from build123d import *

# Parameters (mm, degrees)
SKETCH1_W             = 50.8
SKETCH1_H             = 50.8
BOSS_EXTRUDE1_DEPTH   = 12.7
F_8_CLEARANCE_HOLE1_D = 4.4958
SKETCH5_R             = 13.208
CUT_EXTRUDE1_DEPTH    = 1.5875
SKETCH6_R             = 3.81
CUT_EXTRUDE2_DEPTH    = 39.1
SKETCH10_R            = 6.858
CUT_EXTRUDE3_DEPTH    = 3.175
CUT_EXTRUDE4_START    = -5.334
SKETCH11_R            = 6.858
CUT_EXTRUDE4_DEPTH    = 5.334
SKETCH12_R            = 1.016
CUT_EXTRUDE5_DEPTH    = 19.05
CUT_EXTRUDE6_START    = -19.05
SKETCH13_R            = 1.016
CUT_EXTRUDE6_DEPTH    = 19.05


with BuildPart() as part:
    # Sketch1 → Boss-Extrude1 (new body)
    with BuildSketch(Plane(origin=(0, 0, 0), x_dir=(1, 0, 0), z_dir=(0, 1, 0))):
        Rectangle(SKETCH1_W, SKETCH1_H)
    extrude(amount=BOSS_EXTRUDE1_DEPTH)

    # #8 Clearance Hole1 (through all)
    with Locations(Plane(origin=(0, 12.7, 0), x_dir=(1, 0, 0), z_dir=(0, 1, 0))):
        with Locations((-19.05, -19.05), (-19.05, 19.05), (19.05, 19.05), (19.05, -19.05)):
            Hole(F_8_CLEARANCE_HOLE1_D / 2)

    # Sketch5 → Cut-Extrude1 (cut)
    with BuildSketch(Plane(origin=(0, 12.7, 0), x_dir=(1, 0, 0), z_dir=(0, 1, 0))):
        with Locations(Location((0, 0, 0), (0, 0, 270))):
            Circle(SKETCH5_R)
    extrude(amount=-CUT_EXTRUDE1_DEPTH, mode=Mode.SUBTRACT)

    # Sketch6 → Cut-Extrude2 (cut, through all)
    with BuildSketch(Plane(origin=(0, 12.7, 0), x_dir=(1, 0, 0), z_dir=(0, 1, 0))):
        with Locations(Location((0, 20.32, 0), (0, 0, 270))):
            Circle(SKETCH6_R)
        with Locations(Location((20.32, 0, 0), (0, 0, 270))):
            Circle(SKETCH6_R)
        with Locations(Location((0, -20.32, 0), (0, 0, 270))):
            Circle(SKETCH6_R)
        with Locations(Location((-20.32, 0, 0), (0, 0, 270))):
            Circle(SKETCH6_R)
    extrude(amount=-CUT_EXTRUDE2_DEPTH, mode=Mode.SUBTRACT)

    # Sketch10 → Cut-Extrude3 (cut)
    with BuildSketch(Plane(origin=(0, 12.7, 0), x_dir=(1, 0, 0), z_dir=(0, 1, 0))):
        with Locations((-20.32, 0)):
            Circle(SKETCH10_R)
        with Locations((0, 20.32)):
            Circle(SKETCH10_R)
        with Locations((20.32, 0)):
            Circle(SKETCH10_R)
        with Locations((0, -20.32)):
            Circle(SKETCH10_R)
    extrude(amount=-CUT_EXTRUDE3_DEPTH, mode=Mode.SUBTRACT)

    # Sketch11 → Cut-Extrude4 (cut)
    with BuildSketch(Plane.XZ.offset(CUT_EXTRUDE4_START)):
        with Locations((-20.32, 0)):
            Circle(SKETCH11_R)
        with Locations((0, 20.32)):
            Circle(SKETCH11_R)
        with Locations((20.32, 0)):
            Circle(SKETCH11_R)
        with Locations((0, -20.32)):
            Circle(SKETCH11_R)
    extrude(amount=CUT_EXTRUDE4_DEPTH, mode=Mode.SUBTRACT)

    # Sketch12 → Cut-Extrude5 (cut)
    with BuildSketch(Plane.XY.offset(25.4)):
        with Locations((8.417142715, 9.525)):
            Circle(SKETCH12_R)
    extrude(amount=-CUT_EXTRUDE5_DEPTH, mode=Mode.SUBTRACT)

    # Sketch13 → Cut-Extrude6 (cut)
    with BuildSketch(Plane(origin=(0, 0, -25.4), x_dir=(-1, 0, 0), z_dir=(0, 0, -1)).offset(CUT_EXTRUDE6_START)):
        with Locations(Location((-8.417142715, 9.525, 0), (0, 0, 180))):
            Circle(SKETCH13_R)
    extrude(amount=CUT_EXTRUDE6_DEPTH, mode=Mode.SUBTRACT)


solid = part.part
The model under review builds one solid part; all positions refer to its coordinate system, in mm. A direction names the side the tool comes from. Give positions to 0.01 mm unless a question says otherwise; leave off trailing zeros. Order: outer loops, then holes, each group sorted by start corner. A loop starts at its lowest first (then second) coordinate and runs counter-clockwise, first axis right, second up. Notation, with made-up numbers: M 24,70.25 L 38,70.25 A24 ccw 38,81.25 Z; hole C -4,80.5 d7. An arc over 180 degrees is marked long. Answer in a Markdown table with one row per item. Add a question column.
1. Add section D-D on y = 11.75. State the section outline as (x, z) points, plus the area to 3 significant figures.
2. For pin 1 Ø12.5 at (x, z) = (-20.32, 0) entering from -Y; pin 2 Ø2.5 at (x, z) = (19.05, 19.05) entering from -Y; pin 3 Ø9 at (x, z) = (20.32, 0) entering from +Y (3 decimals); pin 4 Ø1 at (x, y) = (8.5, 10) entering from -Z, all flat-tipped, find the tip position at first contact; note any pin that passes through.
3. Machinability: for faces 4 (the flat face through (8, 10, 6.35)), 5 (the flat face through (-1.62, 9.525, 16.69)), 6 (the cylindrical face through (13.466, 2.704, 0.231)), 7 (the flat face through (8, 10, -6.35)), which of the approach directions +Z, -Z, +X, -X, +Y, -Y give a long, thin tool a straight path to every point of the face, cutting with its end or side? Answer none if there is none.
4. Add section B-B on z = 18. State the section outline as (x, y) points (3 decimals), plus the area to 3 significant figures.
5. Add section C-C on x = 20.32. State the section outline as (y, z) points (3 decimals), plus the area to 3 significant figures.
6. Mouldability with a two-part tool opening along X and no side actions: class faces 1 (the flat face through (25.4, 6, 0)), 2 (the flat face through (0, 6, 25.4)), 3 (the cylindrical face through (9.386, 9.83, 16.008)) as released by +X, released by -X, zero draft, split by the parting line, or undercut.
7. To check wall thickness, follow line 1 along X through (y, z) = (3, -21); line 2 along Z through (x, y) = (19, 8.25); line 3 along X through (y, z) = (10.2, 20.32). State the ranges of each line that lie inside material, in increasing order.
8. Add section A-A on x = 0. Count the separate pieces of the cut face and the enclosed holes in it, plus the area to 3 significant figures.
The answers:
| question | item | result |
|---|---|---|
| 1 | outline | M -25.4,-25.4 L -4.61,-25.4 A6.86 cw long 4.61,-25.4 L 25.4,-25.4 L 25.4,-4.61 A6.86 cw long 25.4,4.61 L 25.4,25.4 L 4.61,25.4 A6.86 cw long -4.61,25.4 L -25.4,25.4 L -25.4,4.61 A6.86 cw long -25.4,-4.61 Z; hole C -19.05,-19.05 d4.5; hole C -19.05,19.05 d4.5; hole C 0,0 d26.42; hole C 19.05,-19.05 d4.5; hole C 19.05,19.05 d4.5 |
| 1 | area | 1,420 mm2 |
| 2 | pin 1 | y = 5.33 |
| 2 | pin 2 | through |
| 2 | pin 3 | y = 9.525 |
| 2 | pin 4 | z = -6.35 |
| 3 | face 4 | +Z |
| 3 | face 5 | +Y |
| 3 | face 6 | -Y |
| 3 | face 7 | -Z |
| 4 | outline | M -25.4,0 L -21.038,0 L -21.038,12.7 L -25.4,12.7 Z; M -17.062,0 L -6.454,0 L -6.454,5.334 L -3.022,5.334 L -3.022,9.525 L -6.454,9.525 L -6.454,12.7 L -17.062,12.7 Z; M 3.022,5.334 L 6.454,5.334 L 6.454,0 L 17.062,0 L 17.062,12.7 L 6.454,12.7 L 6.454,9.525 L 3.022,9.525 Z; M 21.038,0 L 25.4,0 L 25.4,12.7 L 21.038,12.7 Z; hole C 8.417,9.525 d2.032 |
| 4 | area | 406 mm2 |
| 5 | outline | M 0,-25.4 L 12.7,-25.4 L 12.7,-20.905 L 0,-20.905 Z; M 0,-17.195 L 12.7,-17.195 L 12.7,-6.858 L 9.525,-6.858 L 9.525,-3.81 L 5.334,-3.81 L 5.334,-6.858 L 0,-6.858 Z; M 0,6.858 L 5.334,6.858 L 5.334,3.81 L 9.525,3.81 L 9.525,6.858 L 12.7,6.858 L 12.7,17.195 L 0,17.195 Z; M 0,20.905 L 12.7,20.905 L 12.7,25.4 L 0,25.4 Z |
| 5 | area | 402 mm2 |
| 6 | face 1 | released by +X |
| 6 | face 2 | zero draft |
| 6 | face 3 | undercut |
| 7 | line 1 | -25.4 to -20.17, -17.93 to -6.82, 6.82 to 17.93, 20.17 to 25.4 |
| 7 | line 2 | -25.4 to -21.3, -16.8 to -3.57, 3.57 to 16.8, 21.3 to 25.4 |
| 7 | line 3 | -25.4 to -20.9, -17.2 to -6.86, 6.86 to 7.66, 9.18 to 17.2, 20.9 to 25.4 |
| 8 | separate pieces | 3 |
| 8 | enclosed holes | 0 |
| 8 | area | 336 mm2 |
